Geometry check sheet. Reference: the model listing, model coordinates, mm. Face numbers are marked on the shaded views. A direction names the side the tool comes from. Give positions to 0.01 mm unless a question says otherwise; leave off trailing zeros. Write each loop counter-clockwise with the first axis right and the second up, starting at its lowest first coordinate (ties: lowest second). Pieces come first, ordered by that corner, then holes.
(1) Cross-section at A-A (y = 11.5). Count the separate pieces of the cut face and the enclosed holes in it, and give its area (3 significant figures).
(2) Tool access check on the marked faces 1 and 2. Record the directions out of +Z, -Z, +X, -X, +Y, -Y that give a thin tool (end or side, any length) a straight path to the whole face; none if there is none.
(3) Cross-section at D-D (y = 23.25). Record the boundary of the cut face in (x, z), and give its area (3 significant figures).
(4) Thickness scan on line 1 along X through (y, z) = (20, 27); line 2 along Z through (x, y) = (6.5, 19); line 3 along Y through (x, z) = (-9, 21.5). Record the ranges inside material, lowest first.
(5) Cross-section at C-C (x = -9). Record the boundary of the cut face in (y, z), and give its area (3 significant figures).
(6) Mould release check, pull along X, two halves, no side actions. Record for the marked faces 3, 4 and 5: +X half, -X half, draft (parallel to the pull), parting line (faces both ways), or undercut.
(7) Depth check by flat-ended pin: P1, Ø2.5, axis at x = 10.5, z = -31, coming from the +Y side; P2, Ø0.7, axis at y = 11.5, z = -31.5, coming from the -X side; P3, Ø1.8, axis at x = 19, y = 11, coming from the +Z side; P4, Ø2.5, axis at x = 10, z = -31, coming from the -Y side. Enter the tip coordinate at first touch or a pass-through.
(8) Cross-section at B-B (z = 8). Record the boundary of the cut face in (x, y), and give its area (3 significant figures).
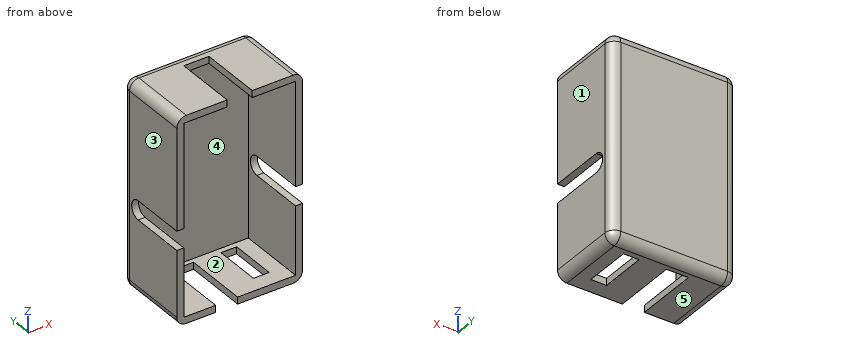
```python
from build123d import *

# Parameters (mm, degrees)
SKETCH2_W           = 40
SKETCH2_H           = 65
SKETCH2_W_2         = 35.6
SKETCH2_H_2         = 60.6
BOSS_EXTRUDE1_DEPTH = 21.85
CUT_EXTRUDE1_DEPTH  = 37.8
SKETCH10_W          = 5
SKETCH10_H          = 15
SKETCH10_W_2        = 7
SKETCH10_H_2        = 20.35
CUT_EXTRUDE2_DEPTH  = 2.2
SKETCH11_W          = 8
SKETCH11_H          = 20
CUT_EXTRUDE3_DEPTH  = 2.2
SKETCH8_W           = 40
SKETCH8_H           = 65
BOSS_EXTRUDE2_DEPTH = 3
FILLET1_R           = 3


with BuildPart() as part:
    # Sketch2 → Boss-Extrude1 (new body)
    with BuildSketch(Plane(origin=(0, 0, 0), x_dir=(-1, 0, 0), z_dir=(0, -1, 0))):
        Rectangle(SKETCH2_W, SKETCH2_H)
        Rectangle(SKETCH2_W_2, SKETCH2_H_2, mode=Mode.SUBTRACT)
    extrude(amount=-BOSS_EXTRUDE1_DEPTH)

    # Sketch9 → Cut-Extrude1 (cut)
    with BuildSketch(Plane(origin=(20, 0, 0), x_dir=(0, 0, -1), z_dir=(1, 0, 0))):
        with BuildLine():
            Line((2.623584384, 17.85), (2.623584384, 0))
            Line((2.623584384, 0), (8.623584384, 0))
            Line((8.623584384, 0), (8.623584384, 17.85))
            ThreePointArc((8.623584384, 17.85), (5.623584384, 20.85), (2.623584384, 17.85))
        make_face()
    cut_extrude1 = extrude(amount=-CUT_EXTRUDE1_DEPTH, mode=Mode.SUBTRACT)

    # Mirror1: Cut-Extrude1 across plane
    add(cut_extrude1.mirror(Plane(origin=(0, 0, 0), x_dir=(0, 0, 1), z_dir=(1, 0, 0))), mode=Mode.SUBTRACT)

    # Sketch10 → Cut-Extrude2 (cut)
    with BuildSketch(Plane(origin=(0, 0, -32.5), x_dir=(-1, 0, 0), z_dir=(0, 0, -1))):
        with Locations((-10.385, 12.57)):
            Rectangle(SKETCH10_W, SKETCH10_H)
        with Locations((4.145, 10.175)):
            Rectangle(SKETCH10_W_2, SKETCH10_H_2)
    extrude(amount=-CUT_EXTRUDE2_DEPTH, mode=Mode.SUBTRACT)

    # Sketch11 → Cut-Extrude3 (cut)
    with BuildSketch(Plane.XY.offset(32.5)):
        with Locations((0, 10)):
            Rectangle(SKETCH11_W, SKETCH11_H)
    extrude(amount=-CUT_EXTRUDE3_DEPTH, mode=Mode.SUBTRACT)

    # Sketch8 → Boss-Extrude2 (add)
    with BuildSketch(Plane(origin=(0, 21.85, 0), x_dir=(1, 0, 0), z_dir=(0, 1, 0))):
        Rectangle(SKETCH8_W, SKETCH8_H)
    extrude(amount=BOSS_EXTRUDE2_DEPTH)

    # Fillet1
    fillet1_edges = [part.edges().sort_by_distance(p)[0] for p in [
        (-20, 12.425, 32.5),
        (20, 12.425, 32.5),
        (20, 12.425, -32.5),
        (-20, 12.425, -32.5),
        (-20, 24.85, 0),
        (0, 24.85, 32.5),
        (20, 24.85, 0),
        (0, 24.85, -32.5),
    ]]
    fillet(fillet1_edges, radius=FILLET1_R)


solid = part.part
```
Reply:
1. separate pieces: 5
1. enclosed holes: 0
1. area: 365 mm2
2. face 1: +Z, -Z, +X, +Y, -Y
2. face 2: -Y
3. outline: (-19.65, -29.5) arc R2.65 ccw to (-17, -32.15) - (17, -32.15) arc R2.65 ccw to (19.65, -29.5) - (19.65, 29.5) arc R2.65 ccw to (17, 32.15) - (-17, 32.15) arc R2.65 ccw to (-19.65, 29.5) - close
3. area: 2,520 mm2
4. line 1: x = -20 to -17.8, 17.8 to 20
4. line 2: z = -32.5 to -30.3, 30.3 to 32.5
4. line 3: y = 21.85 to 24.85
5. outline: (0, -32.5) - (21.85, -32.5) arc R3 ccw to (24.85, -29.5) - (24.85, 29.5) arc R3 ccw to (21.85, 32.5) - (0, 32.5) - (0, 30.3) - (21.85, 30.3) - (21.85, -30.3) - (0, -30.3) - close
5. area: 287 mm2
6. face 3: -X half
6. face 4: undercut
6. face 5: draft
7. P1: stops at y = 24.84
7. P2: stops at x = -19.51
7. P3: stops at z = 32.29
7. P4: stops at y = 0
8. outline: (-20, 0) - (-17.8, 0) - (-17.8, 21.85) - (17.8, 21.85) - (17.8, 0) - (20, 0) - (20, 21.85) arc R3 ccw to (17, 24.85) - (-17, 24.85) arc R3 ccw to (-20, 21.85) - close
8. area: 212 mm2
